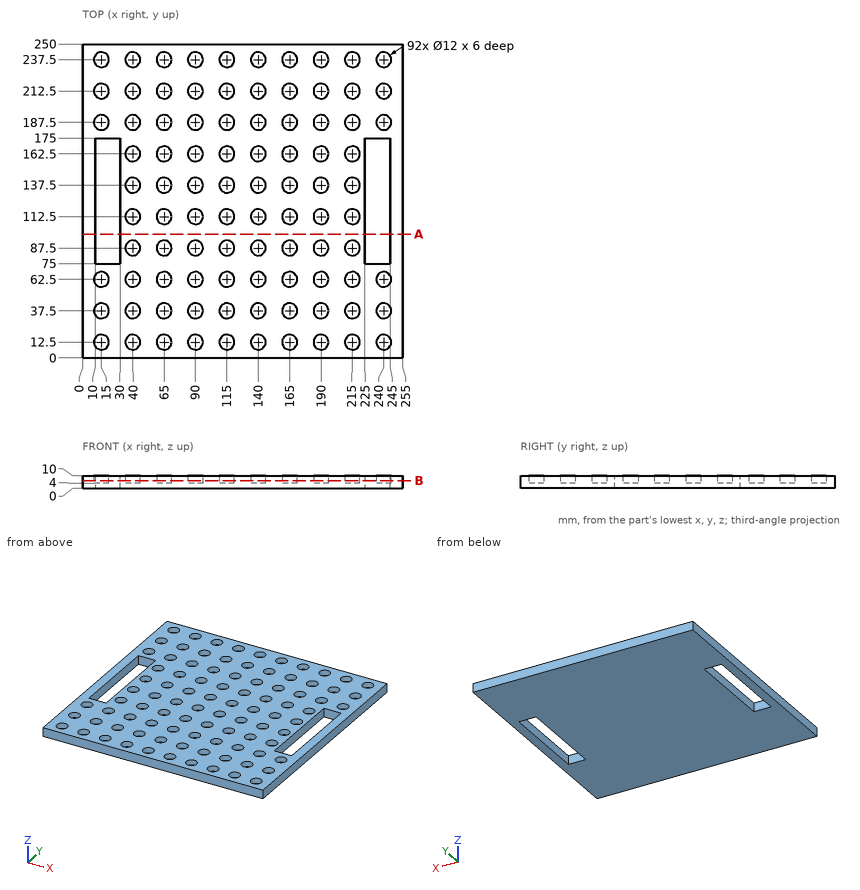
Could you check a few things on this drawing? It's one solid part, dimensions in mm from its lowest x, y, z. Round coordinates to 2 decimals unless told otherwise and drop trailing zeros. Loops run counter-clockwise (first coordinate to the right, second up) from the corner with the lowest first, then second, coordinate; pieces in that order, holes last. Notation, with made-up numbers: M 28.5,89 L 62.5,89 A28 ccw 62.5,109 Z; hole C 85.25,10.25 d10. An arc over 180 degrees is marked long. Write item = value, one per line. Start each with the question number.
(1) I'm going to push a flat-ended pin straight in: P1, Ø3.5, axis at x = 88, y = 215.5, coming from the +Z side. Where does the tip first touch, or does it pass through?
(2) Suppose I cut it at A-A on y = 98.5. Write out the boundary of the cut face in (x, z).
(3) I need wall thicknesses on line 1 along X through (y, z) = (105, 4.5); line 2 along Y through (x, z) = (26, 5); line 3 along Z through (x, y) = (115.5, 236). Which ranges of each line are inside material? Lowest first, please.
(4) Suppose I cut it at B-B on z = 6.25. Give the number of separate pieces and of enclosed holes in the cut face, plus the area to 3 significant figures.
Answer block:
q1.P1 = 4
q2.outline = M 0,0 L 10,0 L 10,10 L 0,10 Z; M 30,0 L 225,0 L 225,10 L 30,10 Z; M 245,0 L 255,0 L 255,10 L 245,10 Z
q3.line_1 = 0 to 10, 30 to 225, 245 to 255
q3.line_2 = 0 to 75, 175 to 250
q3.line_3 = 0 to 4
q4.separate_pieces = 1
q4.enclosed_holes = 94
q4.area = 49,300 mm²
